Part model, mm, in its own coordinate system. Round coordinates to 2 decimals unless told otherwise and drop trailing zeros. Order: outer loops, then holes, each group sorted by start corner. A loop starts at its lowest first (then second) coordinate and runs counter-clockwise, first axis right, second up. Notation, with made-up numbers: (1, 87.5) -> (34, 87.5) arc R25 cw to (34, 116.5) -> close; hole circle Ø3 at (73, -6.75). An arc over 180 degrees is marked (long way). Use CSV: the item, a comma, the result in double quotes.
```python
from build123d import *

# Parameters (mm, degrees)
F0_W     = 225.699038
F0_H     = 159.9
F0_W_2   = 52
F0_H_2   = 34
F0_H_3   = 17
F1_DEPTH = 73


with BuildPart() as f1:
    # F0 (on Front) → F1 (new body)
    with BuildSketch(Plane.XZ):
        with Locations((-274.886772, 47.687937)):
            Rectangle(F0_W, F0_H)
        with Locations((-357.437253, -12.062063)):
            Rectangle(F0_W_2, F0_H_2, mode=Mode.SUBTRACT)
        with Locations((-302.037253, -12.062063)):
            Rectangle(F0_W_2, F0_H_2, mode=Mode.SUBTRACT)
        with Locations((-357.437253, 25.437937)):
            Rectangle(F0_W_2, F0_H_2, mode=Mode.SUBTRACT)
        with Locations((-302.037253, 25.437937)):
            Rectangle(F0_W_2, F0_H_2, mode=Mode.SUBTRACT)
        with Locations((-246.637253, -12.062063)):
            Rectangle(F0_W_2, F0_H_2, mode=Mode.SUBTRACT)
        with Locations((-191.237253, -12.062063)):
            Rectangle(F0_W_2, F0_H_2, mode=Mode.SUBTRACT)
        with Locations((-246.637253, 25.437937)):
            Rectangle(F0_W_2, F0_H_2, mode=Mode.SUBTRACT)
        with Locations((-191.237253, 25.437937)):
            Rectangle(F0_W_2, F0_H_2, mode=Mode.SUBTRACT)
        with Locations((-357.437253, 54.437937)):
            Rectangle(F0_W_2, F0_H_3, mode=Mode.SUBTRACT)
        with Locations((-357.437253, 74.937937)):
            Rectangle(F0_W_2, F0_H_3, mode=Mode.SUBTRACT)
        with Locations((-302.037253, 54.437937)):
            Rectangle(F0_W_2, F0_H_3, mode=Mode.SUBTRACT)
        with Locations((-302.037253, 74.937937)):
            Rectangle(F0_W_2, F0_H_3, mode=Mode.SUBTRACT)
        with Locations((-357.437253, 95.437937)):
            Rectangle(F0_W_2, F0_H_3, mode=Mode.SUBTRACT)
        with Locations((-357.437253, 115.937937)):
            Rectangle(F0_W_2, F0_H_3, mode=Mode.SUBTRACT)
        with Locations((-302.037253, 95.437937)):
            Rectangle(F0_W_2, F0_H_3, mode=Mode.SUBTRACT)
        with Locations((-302.508703, 115.937937)):
            Rectangle(F0_W_2, F0_H_3, mode=Mode.SUBTRACT)
        with Locations((-246.637253, 54.437937)):
            Rectangle(F0_W_2, F0_H_3, mode=Mode.SUBTRACT)
        with Locations((-246.637253, 74.937937)):
            Rectangle(F0_W_2, F0_H_3, mode=Mode.SUBTRACT)
        with Locations((-191.237253, 54.437937)):
            Rectangle(F0_W_2, F0_H_3, mode=Mode.SUBTRACT)
        with Locations((-191.237253, 74.937937)):
            Rectangle(F0_W_2, F0_H_3, mode=Mode.SUBTRACT)
        with Locations((-246.637253, 95.437937)):
            Rectangle(F0_W_2, F0_H_3, mode=Mode.SUBTRACT)
        with Locations((-246.637253, 115.937937)):
            Rectangle(F0_W_2, F0_H_3, mode=Mode.SUBTRACT)
        with Locations((-191.237253, 95.437937)):
            Rectangle(F0_W_2, F0_H_3, mode=Mode.SUBTRACT)
        with Locations((-191.237253, 115.937937)):
            Rectangle(F0_W_2, F0_H_3, mode=Mode.SUBTRACT)
    extrude(amount=F1_DEPTH)


solid = f1.part
```
(1) Cut at B-B, the plane z = 70.5. Give the cut face in (x, y).
Reply:
outline,"(-387.74, -73) -> (-383.44, -73) -> (-383.44, 0) -> (-387.74, 0) -> close; (-331.44, -73) -> (-328.04, -73) -> (-328.04, 0) -> (-331.44, 0) -> close; (-276.04, -73) -> (-272.64, -73) -> (-272.64, 0) -> (-276.04, 0) -> close; (-220.64, -73) -> (-217.24, -73) -> (-217.24, 0) -> (-220.64, 0) -> close; (-165.24, -73) -> (-162.04, -73) -> (-162.04, 0) -> (-165.24, 0) -> close"
(2) Cut at C-C, the plane y = -20.5. State how many separate pieces and enclosed holes the cut face has, then the cut area to 3 significant figures.
Reply:
separate pieces,"1"
enclosed holes,"24"
area,"7,800 mm2"
(3) Cut at A-A, the plane x = -349. Give the cut face in (y, z).
Reply:
outline,"(-73, -32.26) -> (0, -32.26) -> (0, -29.06) -> (-73, -29.06) -> close; (-73, 4.94) -> (0, 4.94) -> (0, 8.44) -> (-73, 8.44) -> close; (-73, 42.44) -> (0, 42.44) -> (0, 45.94) -> (-73, 45.94) -> close; (-73, 62.94) -> (0, 62.94) -> (0, 66.44) -> (-73, 66.44) -> close; (-73, 83.44) -> (0, 83.44) -> (0, 86.94) -> (-73, 86.94) -> close; (-73, 103.94) -> (0, 103.94) -> (0, 107.44) -> (-73, 107.44) -> close; (-73, 124.44) -> (0, 124.44) -> (0, 127.64) -> (-73, 127.64) -> close"
(4) Probe probe 1 along X at (y, z) = (-44.5, 2); probe 2 along X at (y, z) = (-47, 117). List the from-to ranges inside material, lowest first. Write a range as [from, to].
Reply:
probe 1,"[-387.74, -383.44], [-331.44, -328.04], [-276.04, -272.64], [-220.64, -217.24], [-165.24, -162.04]"
probe 2,"[-387.74, -383.44], [-331.44, -328.51], [-276.51, -272.64], [-220.64, -217.24], [-165.24, -162.04]"
